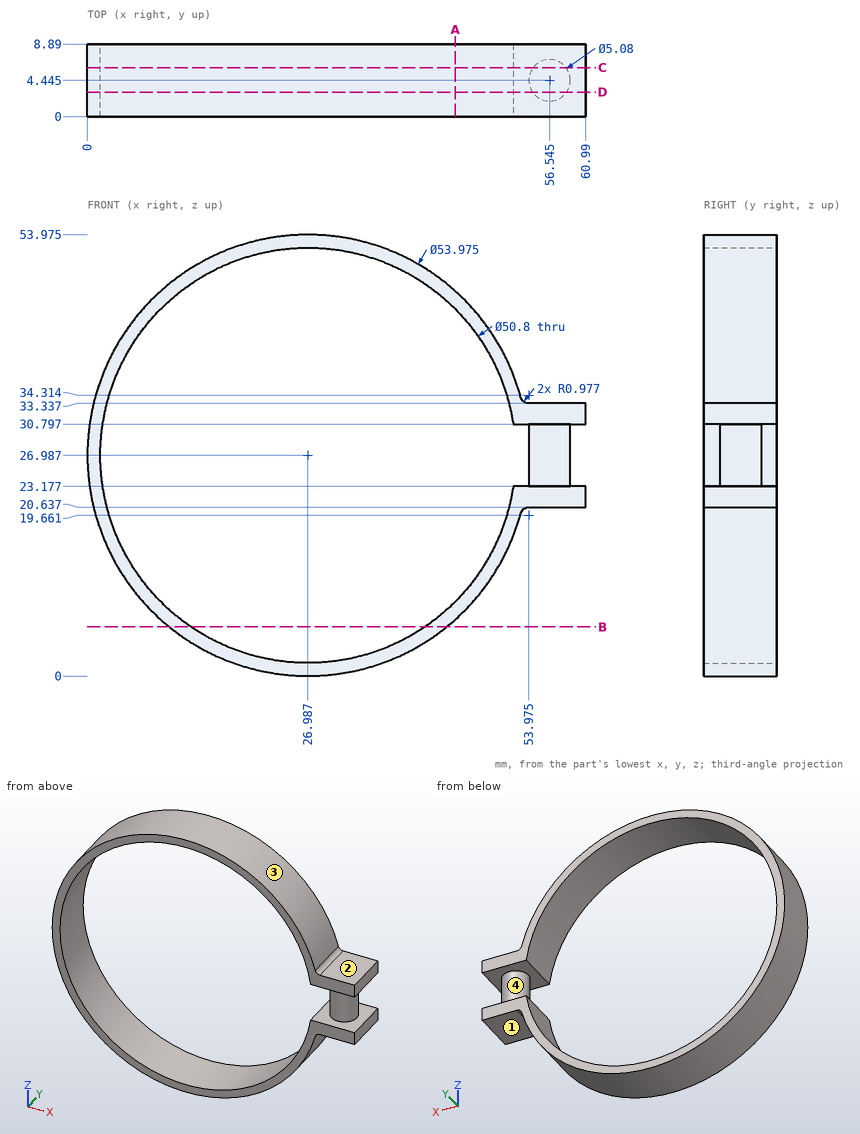
Study the drawing (mm; zero at the part's minimum x, y, z) and answer. Round coordinates to 2 decimals unless told otherwise and drop trailing zeros. Loops run counter-clockwise (first coordinate to the right, second up) from the corner with the lowest first, then second, coordinate; pieces in that order, holes last. Notation, with made-up numbers: M 83.25,-16.5 L 97.25,-16.5 A32 cw 97.25,10.5 Z; hole C 19,11 d1. An arc over 180 degrees is marked long. One line per question, with ' | ' between items.
Q1. The mould has two halves that part along Z. Classify the marked faces 1, 2, 3 and 4: +Z half, -Z half, draft (parallel to the pull), parting line (faces both ways), or undercut.
Conclusion:
face 1: -Z half | face 2: +Z half | face 3: parting line | face 4: undercut
Q2. Find section C-C, the plane y = 6. Give the vertices of the cut face in (x, z) (1 decimal).
Conclusion:
outline: M 53,19.9 A1 cw 54,20.6 L 61,20.6 L 61,23.2 L 58.6,23.2 L 58.6,30.8 L 61,30.8 L 61,33.3 L 54,33.3 A1 cw 53,34.1 A27 ccw long Z; hole M 52.1,23.2 L 54.5,23.2 L 54.5,30.8 L 52.1,30.8 A25.4 ccw long Z
Q3. Find section B-B, the plane z = 6. Give the vertices of the cut face in (x, y) (1 decimal).
Conclusion:
outline: M 10,0 L 12.7,0 L 12.7,8.9 L 10,8.9 Z; M 41.3,0 L 44,0 L 44,8.9 L 41.3,8.9 Z
Q4. Find section A-A, the plane x = 45. Give the vertices of the cut face in (y, z) (1 decimal).
Conclusion:
outline: M 0,6.9 L 8.9,6.9 L 8.9,9.1 L 0,9.1 Z; M 0,44.9 L 8.9,44.9 L 8.9,47.1 L 0,47.1 Z
Q5. Each of these flat-tipped pins is pushed along its axis until it touches: pin 1 Ø1.5 at (x, y) = (15.5, 2) entering from +Z; pin 2 Ø3 at (x, y) = (14, 6.5) entering from +Z; pin 3 Ø3 at (y, z) = (1.5, 22) entering from -X. Where does it stop, or does it pass through?
Conclusion:
pin 1: stops at z = 51.75 | pin 2: stops at z = 51.41 | pin 3: stops at x = 0.23
Q6. Consider line 1 along Z through (x, y) = (54.5, 1.5); line 2 along Z through (x, y) = (18, 5) (1 decimal); line 3 along X through (y, z) = (2.25, 50.5) (1 decimal). Determine where each line is inside the solid, lowest interval first. Write a range as from..to.
Conclusion:
line 1: z = 20.64..23.18, 30.8..33.34 | line 2: z = 1.5..3.2, 50.7..52.4 | line 3: x = 13.7..17.4, 36.6..40.2
